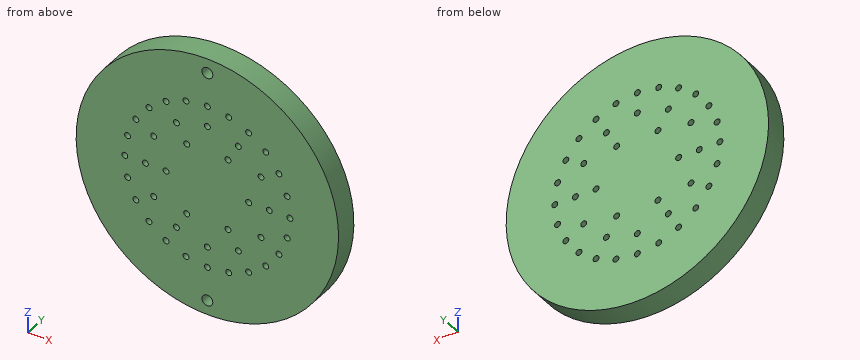
from build123d import *

# Parameters (mm, degrees)
SKETCH1_R             = 28.575
BILLET_DEPTH          = 5.08
SKETCH2_R             = 0.6477
FIRST_LOX_HOLE_DEPTH  = 41.729198985
CIRPATTERN1_COUNT     = 6
CIRPATTERN2_START     = -5.08
CIRPATTERN2_OUTLINE_R = 0.6477
CIRPATTERN2_DEPTH     = 5.08
CIRPATTERN3_START     = -5.08
CIRPATTERN3_OUTLINE_R = 0.6477
CIRPATTERN3_DEPTH     = 5.08
SKETCH4_R             = 1.190625
DOWEL_DEPTH           = 3.175


# Read off the part's stored shape, not the designer's step: CirPattern2, CirPattern3
with BuildPart() as part:
    # Sketch1 → Billet (new body)
    with BuildSketch(Plane(origin=(0, 0, 0), x_dir=(1, 0, 0), z_dir=(0, 1, 0))):
        with Locations(Location((0, 0, 0), (0, 0, 270))):
            Circle(SKETCH1_R)
    extrude(amount=-BILLET_DEPTH)

    # Sketch2 → First Lox Hole (cut, through all)
    with BuildSketch(Plane(origin=(0, 0, 0), x_dir=(1, 0, 0), z_dir=(0, 1, 0))):
        with Locations(Location((8.9916, 0, 0), (0, 0, 270))):
            Circle(SKETCH2_R)
        with Locations(Location((13.4874, 0, 0), (0, 0, 270))):
            Circle(SKETCH2_R)
        with Locations(Location((17.9832, 0, 0), (0, 0, 270))):
            Circle(SKETCH2_R)
    first_lox_hole = extrude(amount=-FIRST_LOX_HOLE_DEPTH, mode=Mode.SUBTRACT)

    # CirPattern1: First Lox Hole ×6 about axis
    cirpattern1_axis = Axis((0, 0, 0), (0, 1, 0))
    for i in range(1, CIRPATTERN1_COUNT):
        add(first_lox_hole.rotate(cirpattern1_axis, i * 360 / CIRPATTERN1_COUNT), mode=Mode.SUBTRACT)

    # CirPattern2 outline → CirPattern2 (cut)
    with BuildSketch(Plane(origin=(0, 0, 0), x_dir=(1, 0, 0), z_dir=(0, 1, 0)).offset(CIRPATTERN2_START)):
        with Locations((11.680431031, -6.7437)):
            Circle(CIRPATTERN2_OUTLINE_R)
        with Locations((0, -13.4874)):
            Circle(CIRPATTERN2_OUTLINE_R)
        with Locations((-11.680431031, -6.7437)):
            Circle(CIRPATTERN2_OUTLINE_R)
        with Locations((-11.680431031, 6.7437)):
            Circle(CIRPATTERN2_OUTLINE_R)
        with Locations((0, 13.4874)):
            Circle(CIRPATTERN2_OUTLINE_R)
        with Locations((11.680431031, 6.7437)):
            Circle(CIRPATTERN2_OUTLINE_R)
    extrude(amount=CIRPATTERN2_DEPTH, mode=Mode.SUBTRACT)

    # CirPattern3 outline → CirPattern3 (cut)
    with BuildSketch(Plane(origin=(0, 0, 0), x_dir=(1, 0, 0), z_dir=(0, 1, 0)).offset(CIRPATTERN3_START)):
        with Locations((17.370437319, -4.654394652)):
            Circle(CIRPATTERN3_OUTLINE_R)
        with Locations((15.573908041, -8.9916)):
            Circle(CIRPATTERN3_OUTLINE_R)
        with Locations((12.716042667, -12.716042667)):
            Circle(CIRPATTERN3_OUTLINE_R)
        with Locations((4.654394652, -17.370437319)):
            Circle(CIRPATTERN3_OUTLINE_R)
        with Locations((0, -17.9832)):
            Circle(CIRPATTERN3_OUTLINE_R)
        with Locations((-4.654394652, -17.370437319)):
            Circle(CIRPATTERN3_OUTLINE_R)
        with Locations((-12.716042667, -12.716042667)):
            Circle(CIRPATTERN3_OUTLINE_R)
        with Locations((-15.573908041, -8.9916)):
            Circle(CIRPATTERN3_OUTLINE_R)
        with Locations((-17.370437319, -4.654394652)):
            Circle(CIRPATTERN3_OUTLINE_R)
        with Locations((-17.370437319, 4.654394652)):
            Circle(CIRPATTERN3_OUTLINE_R)
        with Locations((-15.573908041, 8.9916)):
            Circle(CIRPATTERN3_OUTLINE_R)
        with Locations((-12.716042667, 12.716042667)):
            Circle(CIRPATTERN3_OUTLINE_R)
        with Locations((-4.654394652, 17.370437319)):
            Circle(CIRPATTERN3_OUTLINE_R)
        with Locations((0, 17.9832)):
            Circle(CIRPATTERN3_OUTLINE_R)
        with Locations((4.654394652, 17.370437319)):
            Circle(CIRPATTERN3_OUTLINE_R)
        with Locations((12.716042667, 12.716042667)):
            Circle(CIRPATTERN3_OUTLINE_R)
        with Locations((15.573908041, 8.9916)):
            Circle(CIRPATTERN3_OUTLINE_R)
        with Locations((17.370437319, 4.654394652)):
            Circle(CIRPATTERN3_OUTLINE_R)
    extrude(amount=CIRPATTERN3_DEPTH, mode=Mode.SUBTRACT)

    # Sketch4 → Dowel (cut)
    with BuildSketch(Plane(origin=(0, -5.08, 0), x_dir=(1, 0, 0), z_dir=(0, 1, 0))):
        with Locations(Location((0, 25.4, 0), (0, 0, 270))):
            Circle(SKETCH4_R)
        with Locations(Location((0, -25.4, 0), (0, 0, 90))):
            Circle(SKETCH4_R)
    extrude(amount=DOWEL_DEPTH, mode=Mode.SUBTRACT)


solid = part.part
Verification items for the finished model (mm, model axes). Give positions to 0.01 mm unless a question says otherwise; leave off trailing zeros. Loops run counter-clockwise (first coordinate to the right, second up) from the corner with the lowest first, then second, coordinate; pieces in that order, holes last.
1) Thickness scan on line 1 along X through (y, z) = (-2.9, -6.5); line 2 along Z through (x, y) = (-15.5, -1.7); line 3 along X through (y, z) = (-2.45, -4.5). Record the ranges inside material, lowest first.
2) Sectioned sample at A-A, the plane z = -25. Enter the section's corners in (x, y) (3 decimals), then the cut area to 3 significant figures.
3) Depth check by flat-ended pin: pin 1 Ø3 at (y, z) = (-3.5, 9) entering from +X; pin 2 Ø3 at (x, y) = (-16, -1) entering from -Z; pin 3 Ø1.2 at (x, z) = (0, 25) entering from -Y (3 decimals). Enter the tip coordinate at first touch or a pass-through.
4) Sectioned sample at B-B, the plane x = -23.5. Enter the section's corners in (y, z), then the cut area to 3 significant figures.
5) Sectioned sample at D-D, the plane y = -4.15. Count the separate pieces of the cut face and the enclosed holes in it, then the cut area to 3 significant figures.
6) Sectioned sample at C-C, the plane z = 25.4. Enter the section's corners in (x, y) (3 decimals), then the cut area to 3 significant figures.
Answers:
1. line 1: x = -27.83 to -12.28, -11.08 to 11.08, 12.28 to 27.83
1. line 2: z = -24.01 to -9.64, -8.35 to 8.35, 9.64 to 24.01
1. line 3: x = -28.22 to -18, -16.74 to 16.74, 18 to 28.22
2. outline: (-13.839, -5.08) - (-1.121, -5.08) - (-1.121, -1.905) - (1.121, -1.905) - (1.121, -5.08) - (13.839, -5.08) - (13.839, 0) - (-13.839, 0) - close
2. area: 133 mm2
3. pin 1: stops at x = 27.57
3. pin 2: stops at z = -24.62
3. pin 3: stops at y = -1.905
4. outline: (-5.08, -16.26) - (0, -16.26) - (0, 16.26) - (-5.08, 16.26) - close
4. area: 165 mm2
5. separate pieces: 1
5. enclosed holes: 44
5. area: 2,500 mm2
6. outline: (-13.091, -5.08) - (-1.191, -5.08) - (-1.191, -1.905) - (1.191, -1.905) - (1.191, -5.08) - (13.091, -5.08) - (13.091, 0) - (-13.091, 0) - close
6. area: 125 mm2
